Can you work these out from the model? Positions are in its coordinate system, mm. Round coordinates to 2 decimals unless told otherwise and drop trailing zeros. Order: outer loops, then holes, each group sorted by start corner. A loop starts at its lowest first (then second) coordinate and runs counter-clockwise, first axis right, second up. Notation, with made-up numbers: M 24.25,25 L 83.25,25 A24 cw 83.25,46 Z; hole C 87.25,27.5 d1. An arc over 180 degrees is marked long. Answer as CSV lines item,"result". Start each with the question number.
from build123d import *

# Parameters (mm, degrees)
SKETCH_1_W      = 50
SKETCH_1_H      = 50
EXTRUDE_1_DEPTH = 2000
SKETCH_2_W      = 50
SKETCH_2_H      = 50
EXTRUDE_2_DEPTH = 2000
SKETCH_3_W      = 400
SKETCH_3_H      = 50
EXTRUDE_3_DEPTH = 50
SKETCH_4_W      = 400
SKETCH_4_H      = 50
EXTRUDE_4_DEPTH = 50
SKETCH_5_W      = 400
SKETCH_5_H      = 50
EXTRUDE_5_DEPTH = 50
SKETCH_6_W      = 400
SKETCH_6_H      = 50
EXTRUDE_6_DEPTH = 50
SKETCH_7_W      = 400
SKETCH_7_H      = 50
EXTRUDE_7_DEPTH = 50


with BuildPart() as part:
    # Sketch 1 → Extrude 1 (new body)
    with BuildSketch(Plane.XY):
        with Locations((-200, 0)):
            Rectangle(SKETCH_1_W, SKETCH_1_H)
    extrude(amount=EXTRUDE_1_DEPTH)



with BuildPart() as body_2:
    # Sketch 2 → Extrude 2 (new body)
    with BuildSketch(Plane.XY):
        with Locations((200, 0)):
            Rectangle(SKETCH_2_W, SKETCH_2_H)
    extrude(amount=EXTRUDE_2_DEPTH)


with BuildPart() as part_1:
    add(part.part)

    add(body_2.part)  # Extrude 3 merges body 2
    # Sketch 3 → Extrude 3 (add)
    with BuildSketch(Plane.XY):
        Rectangle(SKETCH_3_W, SKETCH_3_H)
    extrude(amount=EXTRUDE_3_DEPTH)

    # Sketch 4 → Extrude 4 (add)
    with BuildSketch(Plane.XY):
        Rectangle(SKETCH_4_W, SKETCH_4_H)
    extrude(amount=EXTRUDE_4_DEPTH)

    # Sketch 5 → Extrude 5 (add)
    with BuildSketch(Plane.XY):
        Rectangle(SKETCH_5_W, SKETCH_5_H)
    extrude(amount=EXTRUDE_5_DEPTH)

    # Sketch 6 → Extrude 6 (add)
    with BuildSketch(Plane.XY):
        Rectangle(SKETCH_6_W, SKETCH_6_H)
    extrude(amount=EXTRUDE_6_DEPTH)

    # Sketch 7 → Extrude 7 (add)
    with BuildSketch(Plane.XY):
        Rectangle(SKETCH_7_W, SKETCH_7_H)
    extrude(amount=EXTRUDE_7_DEPTH)


solid = part_1.part
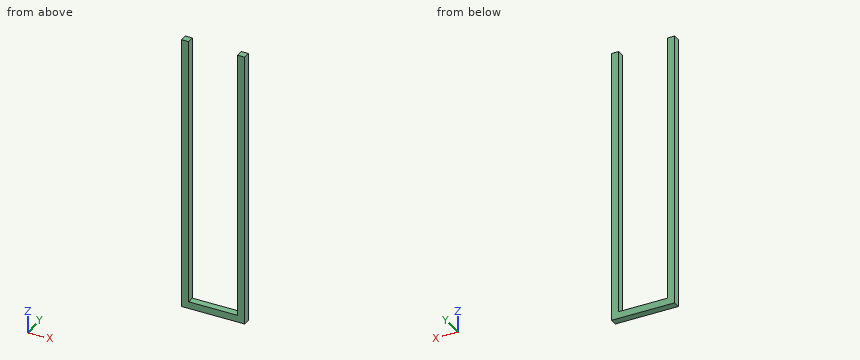
(1) I'm going to push a flat-ended pin straight in: P1, Ø12, axis at x = 152, y = 11.5, coming from the +Z side. Where does the tip first touch, or does it pass through?
(2) I want a section at A-A on z = 1329. Write out the boundary of the cut face in (x, y).
(3) If I drill on line 1 along X through (y, z) = (9, 1781.5); line 2 along Z through (x, y) = (-52.5, -12), over which ranges is the centre line in solid material (lowest first)?
(4) I want a section at C-C on x = 146.5. Write out the boundary of the cut face in (y, z).
(5) I want a section at B-B on y = -7. Write out the boundary of the cut face in (x, z).
From the geometry:
1,P1,"z = 50"
2,outline,"M -225,-25 L -175,-25 L -175,25 L -225,25 Z; M 175,-25 L 225,-25 L 225,25 L 175,25 Z"
3,line 1,"-225 to -175, 175 to 225"
3,line 2,"0 to 50"
4,outline,"M -25,0 L 25,0 L 25,50 L -25,50 Z"
5,outline,"M -225,0 L 225,0 L 225,2000 L 175,2000 L 175,50 L -175,50 L -175,2000 L -225,2000 Z"
